from build123d import *

# Parameters (mm, degrees)
SKETCH_3_W               = 104
SKETCH_3_H               = 58
EXTRUDE_1_DEPTH          = 20
SKETCH_3_R               = 1.5
EXTRUDE_1_2_DEPTH        = 20
EXTRUDE_1_3_DEPTH        = 20
EXTRUDE_1_4_DEPTH        = 20
EXTRUDE_1_5_DEPTH        = 20
SKETCH_4_W               = 104
SKETCH_4_H               = 58
EXTRUDE_2_DEPTH          = 2
EXTRUDE_3_DEPTH          = 3
CUT_EXTRUDE_1_DEPTH      = 118.034964822
CUT_EXTRUDE_1_DEPTH_BACK = 118.034964822
SKETCH_6_R               = 1.5
SKETCH_7_R               = 1.6263635
SKETCH_7_R_2             = 1
EXTRUDE_4_DEPTH          = 5
SKETCH_8_W               = 4
SKETCH_8_H               = 10
CUT_EXTRUDE_2_DEPTH      = 1.274832
SKETCH_9_W               = 4
SKETCH_9_H               = 8
EXTRUDE_5_DEPTH          = 4
SKETCH_11_W              = 4
SKETCH_11_H              = 5.77137
EXTRUDE_7_DEPTH          = 1.82408674
CUT_EXTRUDE_3_REACH      = 123.535
SKETCH_13_W              = 4
SKETCH_13_H              = 8
SKETCH_14_W              = 2
SKETCH_14_H              = 13
EXTRUDE_8_DEPTH          = 2.2
CUT_EXTRUDE_4_REACH      = 123.385
SKETCH_15_W              = 1.5
SKETCH_15_H              = 13
SKETCH_16_W              = 7.456454352
SKETCH_16_H              = 15.223594302
CUT_EXTRUDE_5_DEPTH      = 2


with BuildPart() as part:
    # Sketch 3 → Extrude 1 (new body)
    with BuildSketch(Plane.XY):
        with Locations((49.851592, 26.6635985)):
            Rectangle(SKETCH_3_W, SKETCH_3_H)
        Polygon((97.359934, -0.3), (-0.3, -0.3), (-0.32567, 53.627197), (96.810253, 53.627197), (98.334256, 52.103194), (98.334256, 40.373171), (100.016019, 39.036416919), (100.016019, 4.64681), (98.334516, 2.965177), (98.334516, 0.686792), align=None, mode=Mode.SUBTRACT)
    extrude(amount=EXTRUDE_1_DEPTH)



with BuildPart() as body_2:
    # Sketch 3 → Extrude 1 2 (new body)
    with BuildSketch(Plane.XY):
        with Locations((89.1699285, 50.800132)):
            Circle(SKETCH_3_R)
    extrude(amount=EXTRUDE_1_2_DEPTH)


with BuildPart() as body_3:
    # Sketch 3 → Extrude 1 3 (new body)
    with BuildSketch(Plane.XY):
        with Locations((95.519941, 2.540035)):
            Circle(SKETCH_3_R)
    extrude(amount=EXTRUDE_1_3_DEPTH)


with BuildPart() as body_4:
    # Sketch 3 → Extrude 1 4 (new body)
    with BuildSketch(Plane.XY):
        with Locations((12.970026, 2.540035)):
            Circle(SKETCH_3_R)
    extrude(amount=EXTRUDE_1_4_DEPTH)


with BuildPart() as body_5:
    # Sketch 3 → Extrude 1 5 (new body)
    with BuildSketch(Plane.XY):
        with Locations((14.2448585, 50.793782)):
            Circle(SKETCH_3_R)
    extrude(amount=EXTRUDE_1_5_DEPTH)


with BuildPart() as part_1:
    add(part.part)

    add(body_2.part)  # Extrude 2 merges body 2

    add(body_3.part)  # Extrude 2 merges body 3

    add(body_4.part)  # Extrude 2 merges body 4

    add(body_5.part)  # Extrude 2 merges body 5
    # Sketch 4 → Extrude 2 (add)
    with BuildSketch(Plane(origin=(0, 0, 0), x_dir=(-1, 0, 0), z_dir=(0, 0, -1))):
        with Locations((-49.851592, 26.6635985)):
            Rectangle(SKETCH_4_W, SKETCH_4_H)
    extrude(amount=-EXTRUDE_2_DEPTH)

    # Sketch 5 → Extrude 3 (add)
    with BuildSketch(Plane.XY.offset(2)):
        with BuildLine():
            Line((16.7782735, 50.793782), (16.7782735, 53.627197))
            Line((16.7782735, 53.627197), (11.7114435, 53.627197))
            Line((11.7114435, 53.627197), (11.7114435, 50.793782))
            ThreePointArc((11.7114435, 50.793782), (14.2448585, 48.260367), (16.7782735, 50.793782))
        make_face()
        with BuildLine():
            Line((86.6365135, 50.800132), (86.6365135, 53.633547))
            Line((86.6365135, 53.633547), (91.7033435, 53.633547))
            Line((91.7033435, 53.633547), (91.7033435, 50.800132))
            ThreePointArc((91.7033435, 50.800132), (89.1699285, 48.266717), (86.6365135, 50.800132))
        make_face()
        with BuildLine():
            Line((15.503441, 2.540035), (15.503441, -0.29338))
            Line((15.503441, -0.29338), (10.436611, -0.29338))
            Line((10.436611, -0.29338), (10.436611, 2.540035))
            ThreePointArc((10.436611, 2.540035), (12.970026, 5.07345), (15.503441, 2.540035))
        make_face()
        with BuildLine():
            Line((92.986526, -0.29338), (98.053356, -0.29338))
            Line((98.053356, -0.29338), (98.605799849, -0.29338))
            Line((98.605799849, -0.29338), (100.016019, 4.64681))
            Line((100.016019, 4.64681), (98.334516, 2.965177))
            Line((98.334516, 2.965177), (98.049480092, 2.680119056))
            ThreePointArc((98.049480092, 2.680119056), (95.449872167, 5.072480838), (92.986526, 2.540035))
            Line((92.986526, 2.540035), (92.986526, -0.29338))
        make_face()
    extrude(amount=EXTRUDE_3_DEPTH)

    # Sketch 6 → Cut-Extrude 1 (cut, two sides: drawn at the far end of the back side and taken through both)
    with BuildSketch(Plane.XY.offset(5).offset(-CUT_EXTRUDE_1_DEPTH_BACK)):
        with Locations((14.2448585, 50.793782)):
            Circle(SKETCH_6_R)
        with Locations((89.1699285, 50.800132)):
            Circle(SKETCH_6_R)
        with Locations((12.970026, 2.540035)):
            Circle(SKETCH_6_R)
        with Locations((95.519941, 2.540035)):
            Circle(SKETCH_6_R)
    extrude(amount=CUT_EXTRUDE_1_DEPTH + CUT_EXTRUDE_1_DEPTH_BACK, mode=Mode.SUBTRACT)

    # Sketch 7 → Extrude 4 (add)
    # profile 1 of 4: a face of its own
    with BuildSketch(Plane.XY.offset(5)):
        with Locations((14.2448585, 50.793782)):
            Circle(SKETCH_7_R)
        with Locations((14.2448585, 50.793782)):
            Circle(SKETCH_7_R_2, mode=Mode.SUBTRACT)
    # profile 2 of 4: a face of its own
    with BuildSketch(Plane.XY.offset(5)):
        with Locations((89.1699285, 50.800132)):
            Circle(SKETCH_7_R)
        with Locations((89.1699285, 50.800132)):
            Circle(SKETCH_7_R_2, mode=Mode.SUBTRACT)
    # profile 3 of 4: a face of its own
    with BuildSketch(Plane.XY.offset(5)):
        with Locations((95.519941, 2.540035)):
            Circle(SKETCH_7_R)
        with Locations((95.519941, 2.540035)):
            Circle(SKETCH_7_R_2, mode=Mode.SUBTRACT)
    # profile 4 of 4: a face of its own
    with BuildSketch(Plane.XY.offset(5)):
        with Locations((12.970026, 2.540035)):
            Circle(SKETCH_7_R)
        with Locations((12.970026, 2.540035)):
            Circle(SKETCH_7_R_2, mode=Mode.SUBTRACT)
    extrude(amount=-EXTRUDE_4_DEPTH)

    # Sketch 8 → Cut-Extrude 2 (cut)
    with BuildSketch(Plane(origin=(16.7782735, 0, 0), x_dir=(0, 0, -1), z_dir=(1, 0, 0))):
        with Locations((-8.6, 45.793782)):
            Rectangle(SKETCH_8_W, SKETCH_8_H)
    extrude(amount=-CUT_EXTRUDE_2_DEPTH, mode=Mode.SUBTRACT)

    # Sketch 9 → Extrude 5 (add)
    with BuildSketch(Plane.XY.offset(6.6)):
        with Locations((-2.319669969, 41.022412)):
            Rectangle(SKETCH_9_W, SKETCH_9_H)
    extrude(amount=EXTRUDE_5_DEPTH)

    # Sketch 11 → Extrude 7 (add)
    with BuildSketch(Plane.ZY.offset(2.148408)):
        with Locations((8.6, 47.908097)):
            Rectangle(SKETCH_11_W, SKETCH_11_H)
    extrude(amount=-EXTRUDE_7_DEPTH)

    # Cut-Extrude 3: up to this plane
    cut_extrude_3_end = Plane(origin=(-0.300142736, -0.000142872, 20), z_dir=(-0.9999998867062445, -0.00047601207776012256, 0))
    # Sketch 13 → Cut-Extrude 3 (cut, up to the surface)
    with BuildSketch(Plane.ZY.offset(4.319669969), mode=Mode.PRIVATE) as cut_extrude_3_sk1:
        with Locations((8.6, 41.022412)):
            Rectangle(SKETCH_13_W, SKETCH_13_H)
    cut_extrude_3_tool1 = split(extrude(cut_extrude_3_sk1.sketch, amount=-CUT_EXTRUDE_3_REACH, mode=Mode.PRIVATE), bisect_by=cut_extrude_3_end, keep=Keep.BOTH, mode=Mode.PRIVATE)
    add(cut_extrude_3_tool1.solids().sort_by_distance((-4.31967, 41.022412, 8.6))[0], mode=Mode.SUBTRACT)


with BuildPart() as cut_extrude_3_kept_piece:
    # of the separate pieces the step leaves, the one the design keeps (cut_extrude_3_pieces_kept)
    add(part_1.part.solids().sort_by_distance((-2.148408, -2.3364015, 0))[0])

    # Sketch 14 → Extrude 8 (add)
    with BuildSketch(Plane.XY.offset(5)):
        with Locations((-3.148408, 13.296995)):
            Rectangle(SKETCH_14_W, SKETCH_14_H)
    extrude(amount=EXTRUDE_8_DEPTH)

    # Cut-Extrude 4: up to this plane
    cut_extrude_4_end = Plane(origin=(-0.300142736, -0.000142872, 20), z_dir=(-0.9999998867062445, -0.00047601207776012256, 0))
    # Sketch 15 → Cut-Extrude 4 (cut, up to the surface)
    with BuildSketch(Plane.ZY.offset(4.148408), mode=Mode.PRIVATE) as cut_extrude_4_sk1:
        with Locations((7.95, 13.296995)):
            Rectangle(SKETCH_15_W, SKETCH_15_H)
    cut_extrude_4_tool1 = split(extrude(cut_extrude_4_sk1.sketch, amount=-CUT_EXTRUDE_4_REACH, mode=Mode.PRIVATE), bisect_by=cut_extrude_4_end, keep=Keep.BOTH, mode=Mode.PRIVATE)
    add(cut_extrude_4_tool1.solids().sort_by_distance((-4.148408, 13.296995, 7.95))[0], mode=Mode.SUBTRACT)

    # Sketch 16 → Cut-Extrude 5 (cut)
    with BuildSketch(Plane.ZY.offset(2.148408)):
        with Locations((6.989585085, 13.226446387)):
            Rectangle(SKETCH_16_W, SKETCH_16_H)
    extrude(amount=CUT_EXTRUDE_5_DEPTH, mode=Mode.SUBTRACT)


solid = cut_extrude_3_kept_piece.part
Part model, mm, in its own coordinate system. A direction names the side the tool comes from. Coordinates: 2 decimals unless noted, no trailing zeros. Order: outer loops, then holes, each group sorted by start corner. A loop starts at its lowest first (then second) coordinate and runs counter-clockwise, first axis right, second up. Notation, with made-up numbers: M -3,35.5 L 16,35.5 A13 ccw 16,49.5 Z; hole C 36,48 d4. An arc over 180 degrees is marked long. Use a Markdown table: item, result.
(1) Cut at D-D on y = 15. Write the cut outline in (x, z), then the cut area to 3 significant figures.
A:
| item | result |
|---|---|
| outline | M -2.15,0 L 101.85,0 L 101.85,20 L 100.02,20 L 100.02,2 L -0.31,2 L -0.31,7.2 L -2.15,7.2 Z; M -2.15,8.7 L -0.31,8.7 L -0.31,20 L -2.15,20 Z |
| area | 271 mm^2 |
(2) Cut at C-C on z = 13.5. Write the cut outline in (x, y).
A:
| item | result |
|---|---|
| outline | M -2.15,-2.34 L 101.85,-2.34 L 101.85,55.66 L -2.15,55.66 Z; hole M -0.33,53.63 L -0.3,-0.3 L 97.36,-0.3 L 98.33,0.69 L 98.33,2.97 L 100.02,4.65 L 100.02,39.04 L 98.33,40.37 L 98.33,52.1 L 96.81,53.63 Z |
(3) Pull direction X, two halves, no side cores. Call faces 1 (the flat face through (51, 27, 2)), 2 (the flat face through (49, 55.664, 10)), 3 (the flat face through (101.852, 26, 10)): released by +X, released by -X, zero draft, split by the parting line, or undercut.
A:
| item | result |
|---|---|
| face 1 | undercut |
| face 2 | zero draft |
| face 3 | released by +X |
(4) Flat gauge pins, fed straight in: pin 1 (6 mm diameter, centred on x = 94.5, y = 3.5, fed in from +Z); pin 2 (6 mm diameter, centred on x = 43, y = 22, fed in from -Z). Where does each tip first touch, or does it go through?
A:
| item | result |
|---|---|
| pin 1 | stops at z = 5 |
| pin 2 | stops at z = 0 |
(5) Cut at B-B on x = 32.5. Write the cut outline in (y, z).
A:
| item | result |
|---|---|
| outline | M -2.34,0 L 55.66,0 L 55.66,20 L 53.63,20 L 53.63,2 L -0.3,2 L -0.3,20 L -2.34,20 Z |
(6) Cut at A-A on y = 42. Write the cut outline in (x, z), then the cut area to 3 significant figures.
A:
| item | result |
|---|---|
| outline | M -2.15,0 L 101.85,0 L 101.85,20 L 98.33,20 L 98.33,2 L -0.32,2 L -0.32,6.6 L -2.15,6.6 Z; M -2.15,10.6 L -0.32,10.6 L -0.32,20 L -2.15,20 Z |
| area | 297 mm^2 |
(7) Probe L1, parallel to X at y = 30, z = 10; L2, parallel to X at y = 49.5, z = 14; L3, parallel to Y at x = 44, z = 8.5. List the from-to ranges inside material, lowest first.
A:
| item | result |
|---|---|
| L1 | x = -2.15 to -0.31, 100.02 to 101.85 |
| L2 | x = -2.15 to -0.32, 98.33 to 101.85 |
| L3 | y = -2.34 to -0.3, 53.63 to 55.66 |
(8) Tool access for faces 4 (the cylindrical face through (11.97, 2.58, 2.54)), 5 (the flat face through (98.335, 2, 12)), 6 (the flat face through (-1, 45.022, 9)): list every direction of +Z, -Z, +X, -X, +Y, -Y with a clear straight run to the whole face (end or side of a thin tool).
A:
| item | result |
|---|---|
| face 4 | +Z, -Z |
| face 5 | +Z |
| face 6 | -X |
